Check sheet for the modelled part. Datum: model origin and axes. Units: mm. Face numbers are marked on the shaded views. A direction names the side the tool comes from. Coordinates: 2 decimals unless noted, no trailing zeros. Loops run counter-clockwise (first coordinate to the right, second up) from the corner with the lowest first, then second, coordinate; pieces in that order, holes last. Notation, with made-up numbers: (-16.5, 65) - (9.5, 65) arc R15 ccw to (9.5, 72) - close; hole circle Ø9 at (68, -26.75). An arc over 180 degrees is marked (long way). Write each question's results on one line, items separated by ' | '. Start each with the question number.
1. Cross-section at A-A (x = -4). Record the cut outline in (y, z), and give its area (3 significant figures).
2. Tool access check on the marked faces 5 and 6. Record the directions out of +Z, -Z, +X, -X, +Y, -Y that give a thin tool (end or side, any length) a straight path to the whole face; none if there is none.
3. Draft check along X on the marked faces 1, 2, 3 and 4. Enter one of: released by +X, released by -X, zero draft, split by the parting line, or undercut.
4. Cross-section at D-D (x = -23.5). Record the cut outline in (y, z), and give its area (3 significant figures).
5. Gauge pin test, flat ends, axial feed: P1, Ø1.4, axis at x = -4, z = -4.62, coming from the +Y side; P2, Ø2.5, axis at x = -4.5, z = -4.5, coming from the -Y side; P3, Ø2, axis at x = -26.5, z = -34, coming from the -Y side. Record the tip position at first contact, or that the pin passes through.
6. Thickness scan on line 1 (Z direction, x = -22, y = -0.65); line 2 (Z direction, x = -4, y = 1.2); line 3 (X direction, y = -0.05, z = -33). Record the ranges inside material, lowest first. Write a range as [from, to].
Autodesk Inventor part; units mm, degrees
ref_plane "YZ Plane" through (0, 0, 0) normal (1, 0, 0) x (0, 1, 0)
ref_plane "XZ Plane" through (0, 0, 0) normal (0, 1, 0) x (-1, 0, 0)
ref_plane "XY Plane" through (0, 0, 0) normal (0, 0, 1) x (1, 0, 0)
sketch "スケッチ1" plane through (0, 0, 0) normal (0, 1, 0) x (-1, 0, 0)
  line L0 (26, 0) -> (0, 0)
  line L1 (0, 0) -> (0, -30)
  line L2 (0, -30) -> (26, -30)
  line L3 (26, -30) -> (26, 0)
  line L4 (26, 0) -> (27.9445, -37.1034)
  line L5 (0, 0) -> (-1.9445, -37.1034)
  arc A0 (-1.9445, -37.1034) -> (27.9445, -37.1034) centre (13, 0) ccw
  line L6 (0, 0) -> (26, -30)
  line L7 (0, -30) -> (26, 0)
  line L8 (4, -4.6154) -> (22, -4.6154)
  line L9 (22, -4.6154) -> (22, -25.3846)
  line L10 (22, -25.3846) -> (4, -25.3846)
  line L11 (4, -25.3846) -> (4, -4.6154)
  circle A1 centre (4, -4.6154) radius 0.8
  circle A2 centre (4, -25.3846) radius 0.8
  circle A3 centre (22, -4.6154) radius 0.8
  circle A4 centre (22, -25.3846) radius 0.8
  line L12 (38, 0) -> (-12, 0)
  line L13 (-12, 0) -> (-12, -40)
  line L14 (-12, -40) -> (38, -40)
  line L15 (38, -40) -> (38, 0)
  point P0 (13, -40)
  point P1 (13, -40)
  dimension "d0" = 26
  dimension "d3" = 30
  dimension "d4" = 3
  dimension "d5" = 3
  dimension "d6" = 40
  dimension "d17" = 4
  dimension "d18" = 1.6
  dimension "d19" = 1.6
  dimension "d20" = 1.6
  dimension "d21" = 1.6
  dimension "d28" = 50
extrude "押し出し1" add sketch "スケッチ1" along normal blind 4 contours L7 A3 L8 A1 L6 L0 | L4 A0 L5 L1 L2 L3 | L12 L15 L14 A0 L4 | L3 L6 A4 L9 A3 L7 | L6 A1 L11 A2 L7 L1 | L5 A0 L14 L13 L12 | L2 L7 A2 L10 A4 L6 | A3 L7 L6 A1 L8 | A1 L6 L7 A2 L11 | L10 A2 L7 L6 A4 | A3 L9 A4 L6 L7
sketch "スケッチ4" plane through (0, 0, 0) normal (0, -1, 0) x (1, 0, 0)
  line L0 (-38, 0) -> (12, 0)
  line L1 (-38, -40) -> (-38, 0)
  line L2 (12, -40) -> (-38, -40)
  line L3 (12, 0) -> (12, -40)
  circle A0 centre (-4, -25.3846) radius 0.8
  circle A1 centre (-22, -25.3846) radius 0.8
  circle A2 centre (-4, -4.6154) radius 0.8
  circle A3 centre (-22, -4.6154) radius 0.8
  circle A4 centre (-22, -4.6154) radius 2.5
  circle A5 centre (-4, -4.6154) radius 2.5
  circle A6 centre (-4, -25.3846) radius 2.5
  circle A7 centre (-22, -25.3846) radius 2.5
  line L4 (-36, -8) -> (-26, -8)
  line L5 (-26, -8) -> (-26, -38)
  line L6 (-26, -38) -> (-36, -38)
  line L7 (-36, -38) -> (-36, -8)
  line L8 (0, -8) -> (10, -8)
  line L9 (10, -8) -> (10, -38)
  line L10 (10, -38) -> (0, -38)
  line L11 (0, -38) -> (0, -8)
  point P0 (0, 0)
  dimension "d29" = 5
  dimension "d32" = 10
  dimension "d33" = 30
  dimension "d34" = 10
  dimension "d35" = 30
  dimension "d36" = 2
  dimension "d37" = 2
  dimension "d38" = 2
extrude "押し出し5" add sketch "スケッチ4" along normal blind 1 contours L0 L3 L2 L1
fillet "フィレット3" radius 1 8 edges at (-31, -1, -8) (-26, -1, -23) (-31, -1, -38) (-36, -1, -23) (0, -1, -23) (10, -1, -23) (5, -1, -8) (5, -1, -38)
properties part number "toe_sole_back"
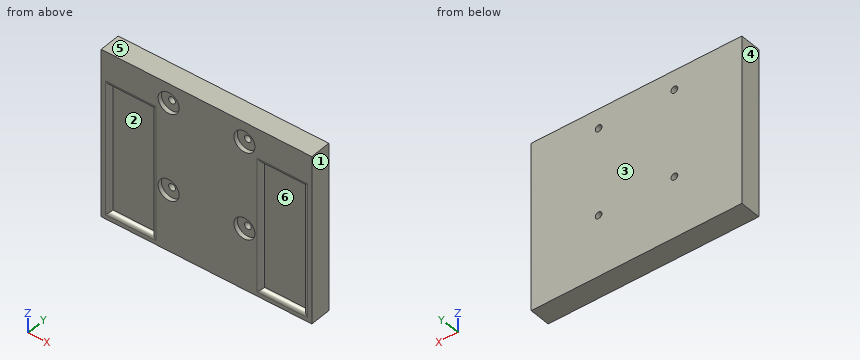
Established:
1) outline: (-1, -40) - (4, -40) - (4, -26.18) - (0, -26.18) - (0, -27.88) - (-1, -27.88) - close; (-1, -22.88) - (0, -22.88) - (0, -24.58) - (4, -24.58) - (4, -5.42) - (0, -5.42) - (0, -7.12) - (-1, -7.12) - close; (-1, -2.12) - (0, -2.12) - (0, -3.82) - (4, -3.82) - (4, 0) - (-1, 0) - close | area: 177 mm^2
2) face 5: +Z, +X, -X, +Y, -Y | face 6: -Y
3) face 1: released by +X | face 2: undercut | face 3: zero draft | face 4: released by -X
4) outline: (-1, -40) - (4, -40) - (4, 0) - (-1, 0) - (-1, -2.62) - (0, -2.62) - (0, -6.62) - (-1, -6.62) - (-1, -23.38) - (0, -23.38) - (0, -27.38) - (-1, -27.38) - close | area: 192 mm^2
5) P1: through | P2: y = 0 | P3: y = -0.87
6) line 1: [-40, -27.88], [-22.88, -7.12], [-2.12, 0] | line 2: [-40, -26.18], [-24.58, -5.42], [-3.82, 0] | line 3: [-38, -36], [-26, 0], [10, 12]
